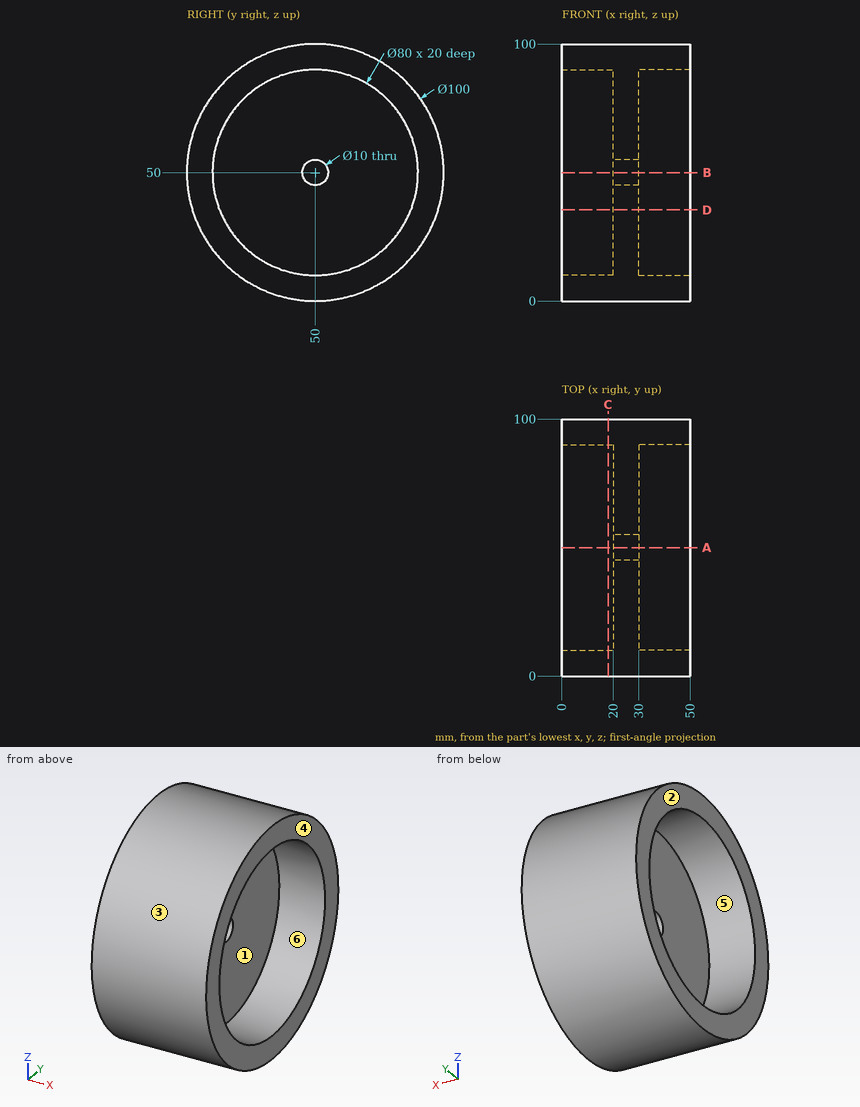
The figure shows three views and two pictorial views of one solid part (mm, origin at its lowest corner). Answer the questions. A direction names the side the tool comes from. Give positions to 0.01 mm unless a question says otherwise; leave off trailing zeros. Write each loop counter-clockwise with the first axis right and the second up, starting at its lowest first coordinate (ties: lowest second). Pieces come first, ordered by that corner, then holes. Notation, with made-up numbers: (-36, 33.5) -> (0, 33.5) arc R13 cw to (0, 52.5) -> close; hole circle Ø4 at (56.5, 43.25). An arc over 180 degrees is marked (long way). Answer as a JSON object with one key per item and string values.
1) Section D-D on z = 35.5 is taken. Write down the section's boundary in (x, y).
Findings below:
{"outline": "(0, 2.15) -> (50, 2.15) -> (50, 12.72) -> (30, 12.72) -> (30, 87.28) -> (50, 87.28) -> (50, 97.85) -> (0, 97.85) -> (0, 87.28) -> (20, 87.28) -> (20, 12.72) -> (0, 12.72) -> close"}
2) A tool of negligible diameter and unlimited length cuts with its end or side. For the marked faces 4, 5 and 6, from which of +Z, -Z, +X, -X, +Y, -Y can it reach the whole face along a straight path? Write none if from no direction.
Findings below:
{"face 4": "+Z, -Z, +X, +Y, -Y", "face 5": "-X", "face 6": "+X"}
3) Straight lines are drawn through the part: probe 1 along Y at (x, z) = (44.25, 50); probe 2 along Y at (x, z) = (24, 50); probe 3 along Z at (x, y) = (7, 73). For each, find the intervals that lie inside material, in ascending order. Write a range as from..to.
Findings below:
{"probe 1": "y = 0..10, 90..100", "probe 2": "y = 0..45, 55..100", "probe 3": "z = 5.6..17.27, 82.73..94.4"}
4) Flat-ended cylindrical pins translate along their axes: pin 1 Ø10 at (x, y) = (12.5, 37) entering from +Z; pin 2 Ø10 at (x, y) = (26.5, 73) entering from +Z; pin 3 Ø2 at (x, y) = (28, 14) entering from -Z. Find the tip coordinate at first contact, or state that the pin passes through.
Findings below:
{"pin 1": "stops at z = 99.36", "pin 2": "stops at z = 96.65", "pin 3": "stops at z = 14.29"}
5) Section A-A on y = 50 is taken. Write down the section's boundary in (x, z).
Findings below:
{"outline": "(0, 0) -> (50, 0) -> (50, 10) -> (30, 10) -> (30, 45) -> (20, 45) -> (20, 10) -> (0, 10) -> close; (0, 90) -> (20, 90) -> (20, 55) -> (30, 55) -> (30, 90) -> (50, 90) -> (50, 100) -> (0, 100) -> close"}
6) Section C-C on x = 18 is taken. Write down the section's boundary in (y, z), then the cut area to 3 significant figures.
Findings below:
{"outline": "circle Ø100 at (50, 50); hole circle Ø80 at (50, 50)", "area": "2,830 mm^2"}
7) For a pull along Z with two mould halves and no side action, classify the marked faces 1, 2 and 3 as pulls with the +Z half, pulls with the -Z half, needs draft (parallel to the pull), parting line crosses it, or undercut.
Findings below:
{"face 1": "undercut", "face 2": "needs draft", "face 3": "parting line crosses it"}
